Geometry: see drawing. Coordinates: mm, zero at the bounding-box minimum. A direction names the side the tool comes from. Coordinates: 2 decimals unless noted, no trailing zeros. Order: outer loops, then holes, each group sorted by start corner. A loop starts at its lowest first (then second) coordinate and runs counter-clockwise, first axis right, second up.
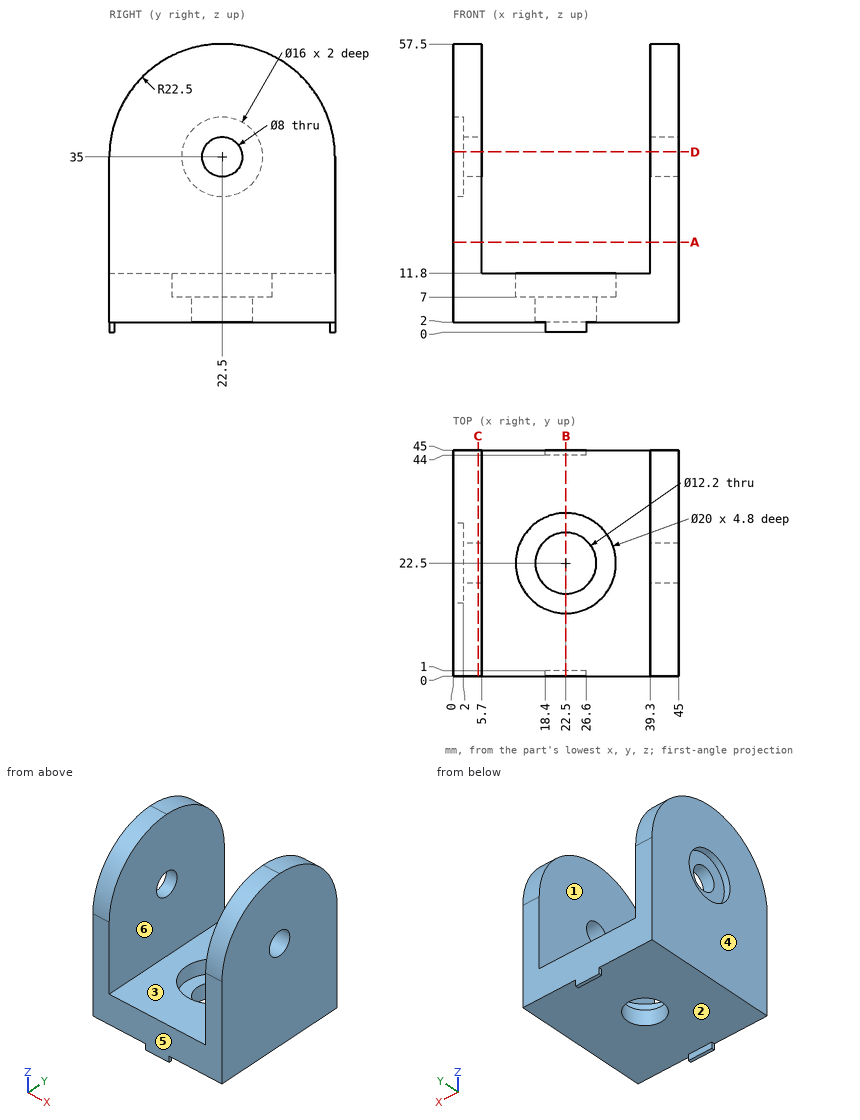
Q1. Section query A-A on z = 18. Output: boundary loops of the cut face in (x, y).
Solutions:
outline: (0, 0) - (5.7, 0) - (5.7, 45) - (0, 45) - close; (39.3, 0) - (45, 0) - (45, 45) - (39.3, 45) - close
Q2. Section query D-D on z = 36. Output: boundary loops of the cut face in (x, y), plus the area to 3 significant figures.
Solutions:
outline: (0, 0.02) - (5.7, 0.02) - (5.7, 18.63) - (2, 18.63) - (2, 14.56) - (0, 14.56) - close; (0, 30.44) - (2, 30.44) - (2, 26.37) - (5.7, 26.37) - (5.7, 44.98) - (0, 44.98) - close; (39.3, 0.02) - (45, 0.02) - (45, 18.63) - (39.3, 18.63) - close; (39.3, 26.37) - (45, 26.37) - (45, 44.98) - (39.3, 44.98) - close
area: 408 mm2
Q3. Material intervals for line 1 along Y through (x, z) = (42.4, 35); line 2 along X through (y, z) = (15.5, 12); line 3 along Z through (x, y) = (33.5, 28), sorted ascending.
Solutions:
line 1: y = 0 to 18.5, 26.5 to 45
line 2: x = 0 to 5.7, 39.3 to 45
line 3: z = 2 to 11.8
Q4. Set-up query: the marked faces 5 and 6. Return all of +Z, -Z, +X, -X, +Y, -Y with unobstructed straight access to the full face (end or side cutting, diameter ignored); none if empty.
Solutions:
face 5: +Z, -Z, +X, -X, -Y
face 6: +Z, +Y, -Y
Q5. Section query C-C on x = 5. Output: boundary loops of the cut face in (y, z).
Solutions:
outline: (0, 2) - (45, 2) - (45, 35) arc R22.5 ccw to (0, 35) - close; hole circle Ø8 at (22.5, 35)
Q6. Pin query (flat end, axial travel): P1, Ø0.8, axis at y = 44.5, z = 0.5, coming from the -X side; P2, Ø1.6, axis at x = 21, z = 1, coming from the -Y side; P3, Ø10, axis at x = 19, y = 25.5, coming from the +Z side; P4, Ø1, axis at x = 35.5, y = 18.5, coming from the -Z side. Return the tip coordinate at first contact, or that it passes through.
Solutions:
P1: stops at x = 18.4
P2: stops at y = 0
P3: stops at z = 7
P4: stops at z = 2
Q7. Pull-direction query (X, two-part tool) for the marked faces 1, 2, 3 and 4; classes: pulls with the +X half, pulls with the -X half, needs draft (parallel to the pull), parting line crosses it, or undercut.
Solutions:
face 1: undercut
face 2: needs draft
face 3: undercut
face 4: pulls with the -X half
Q8. Section query B-B on x = 22.5. Output: boundary loops of the cut face in (y, z), plus the area to 3 significant figures.
Solutions:
outline: (0, 0) - (1, 0) - (1, 2) - (16.4, 2) - (16.4, 7) - (12.5, 7) - (12.5, 11.8) - (0, 11.8) - close; (28.6, 2) - (44, 2) - (44, 0) - (45, 0) - (45, 11.8) - (32.5, 11.8) - (32.5, 7) - (28.6, 7) - close
area: 288 mm2
